Check sheet for the drawn part. Datum: minimum x, y, z corner. Units: mm. Round coordinates to 2 decimals unless told otherwise and drop trailing zeros. Write each loop counter-clockwise with the first axis right and the second up, starting at its lowest first coordinate (ties: lowest second). Pieces come first, ordered by that corner, then holes. Notation, with made-up numbers: (-35.5, 30) -> (-12.5, 30) arc R29 ccw to (-12.5, 61) -> close; hole circle Ø5 at (17.25, 13.5). An arc over 180 degrees is marked (long way). One line per item, written item: value. Start each with the question number.
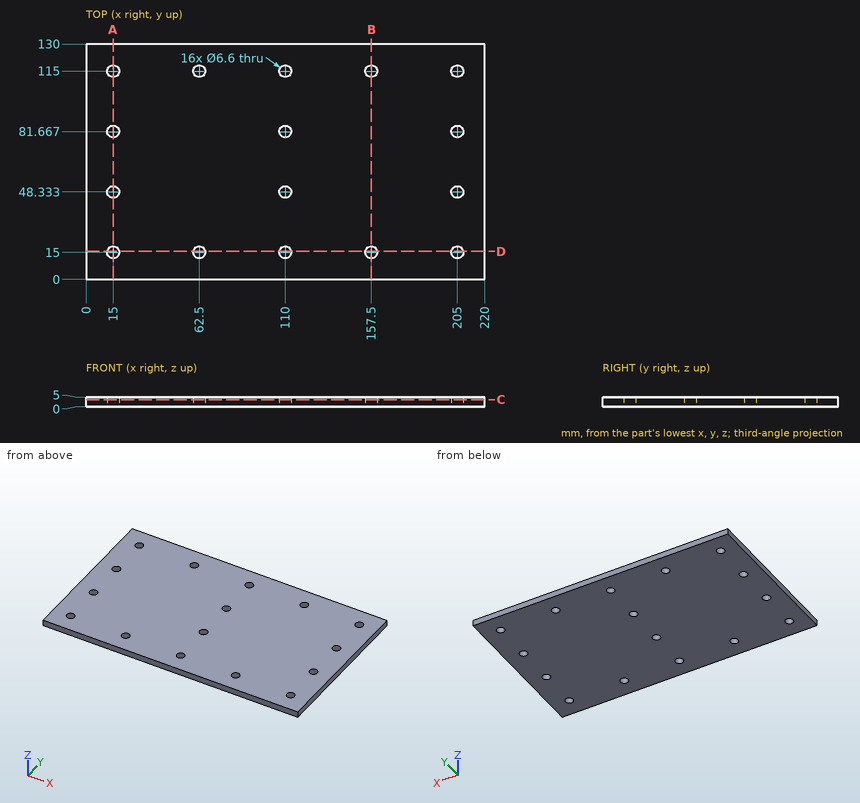
1. Cross-section at A-A (x = 15). Record the cut outline in (y, z), plus the area to 3 significant figures.
2. Cross-section at C-C (z = 3.75). Give the number of separate pieces and of enclosed holes in the cut face, plus the area to 3 significant figures.
3. Material ranges on probe 1 along X at (y, z) = (115, 3.3); probe 2 along Y at (x, z) = (110, 3.9); probe 3 along X at (y, z) = (51, 2.15) (1 decimal), recorded low to high.
4. Cross-section at B-B (x = 157.5). Record the cut outline in (y, z).
5. Cross-section at D-D (y = 15.5). Record the cut outline in (x, z), plus the area to 3 significant figures.
Working result:
1. outline: (0, 0) -> (11.7, 0) -> (11.7, 5) -> (0, 5) -> close; (18.3, 0) -> (45.03, 0) -> (45.03, 5) -> (18.3, 5) -> close; (51.63, 0) -> (78.37, 0) -> (78.37, 5) -> (51.63, 5) -> close; (84.97, 0) -> (111.7, 0) -> (111.7, 5) -> (84.97, 5) -> close; (118.3, 0) -> (130, 0) -> (130, 5) -> (118.3, 5) -> close
1. area: 518 mm^2
2. separate pieces: 1
2. enclosed holes: 16
2. area: 28,100 mm^2
3. probe 1: x = 0 to 11.7, 18.3 to 59.2, 65.8 to 106.7, 113.3 to 154.2, 160.8 to 201.7, 208.3 to 220
3. probe 2: y = 0 to 11.7, 18.3 to 45.03, 51.63 to 78.37, 84.97 to 111.7, 118.3 to 130
3. probe 3: x = 0 to 13.1, 16.9 to 108.1, 111.9 to 203.1, 206.9 to 220
4. outline: (0, 0) -> (11.7, 0) -> (11.7, 5) -> (0, 5) -> close; (18.3, 0) -> (111.7, 0) -> (111.7, 5) -> (18.3, 5) -> close; (118.3, 0) -> (130, 0) -> (130, 5) -> (118.3, 5) -> close
5. outline: (0, 0) -> (11.74, 0) -> (11.74, 5) -> (0, 5) -> close; (18.26, 0) -> (59.24, 0) -> (59.24, 5) -> (18.26, 5) -> close; (65.76, 0) -> (106.74, 0) -> (106.74, 5) -> (65.76, 5) -> close; (113.26, 0) -> (154.24, 0) -> (154.24, 5) -> (113.26, 5) -> close; (160.76, 0) -> (201.74, 0) -> (201.74, 5) -> (160.76, 5) -> close; (208.26, 0) -> (220, 0) -> (220, 5) -> (208.26, 5) -> close
5. area: 937 mm^2
